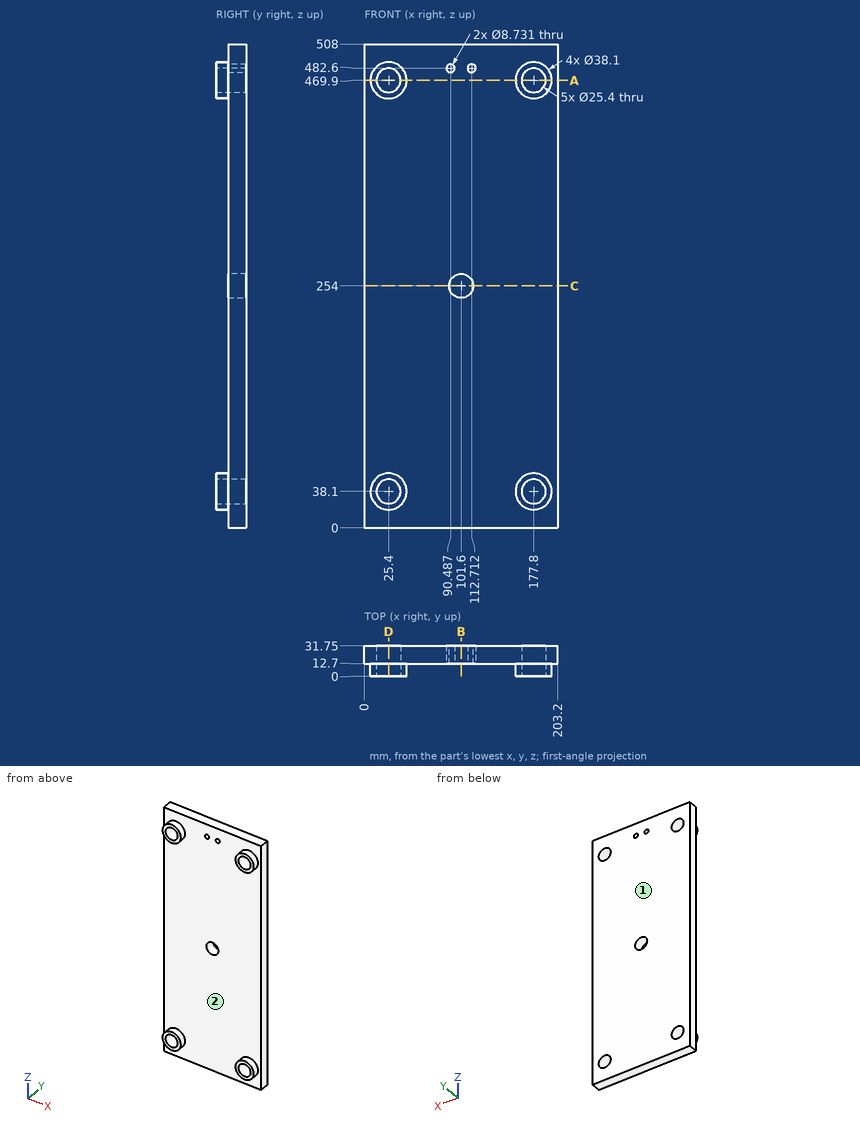
The drawing under review shows one solid part. Ordinate dimensions are in mm from its lowest x, y, z. Round coordinates to 2 decimals unless told otherwise and drop trailing zeros. Loops run counter-clockwise (first coordinate to the right, second up) from the corner with the lowest first, then second, coordinate; pieces in that order, holes last. Notation, with made-up numbers: (-39.75, 11.5) - (-3.75, 11.5) arc R24 cw to (-3.75, 27.5) - close; hole circle Ø11 at (85.25, 67.5). An arc over 180 degrees is marked (long way). One line per question, with ' | ' between items.
1. We need section D-D, the plane x = 25.4. State the section outline as (y, z) points, and give its area (3 significant figures).
Results are:
outline: (0, 19.05) - (12.7, 19.05) - (12.7, 0) - (31.75, 0) - (31.75, 25.4) - (0, 25.4) - close; (0, 50.8) - (31.75, 50.8) - (31.75, 457.2) - (0, 457.2) - (0, 450.85) - (12.7, 450.85) - (12.7, 57.15) - (0, 57.15) - close; (0, 482.6) - (31.75, 482.6) - (31.75, 508) - (12.7, 508) - (12.7, 488.95) - (0, 488.95) - close | area: 9,030 mm²
2. We need section A-A, the plane z = 469.9. State the section outline as (x, y) points.
Results are:
outline: (0, 12.7) - (6.35, 12.7) - (6.35, 0) - (12.7, 0) - (12.7, 31.75) - (0, 31.75) - close; (38.1, 0) - (44.45, 0) - (44.45, 12.7) - (158.75, 12.7) - (158.75, 0) - (165.1, 0) - (165.1, 31.75) - (38.1, 31.75) - close; (190.5, 0) - (196.85, 0) - (196.85, 12.7) - (203.2, 12.7) - (203.2, 31.75) - (190.5, 31.75) - close
3. We need section B-B, the plane x = 101.6. State the section outline as (y, z) points.
Results are:
outline: (12.7, 0) - (31.75, 0) - (31.75, 241.3) - (12.7, 241.3) - close; (12.7, 266.7) - (31.75, 266.7) - (31.75, 508) - (12.7, 508) - close
4. We need section C-C, the plane z = 254. State the section outline as (x, y) points, and give its area (3 significant figures).
Results are:
outline: (0, 12.7) - (88.9, 12.7) - (88.9, 31.75) - (0, 31.75) - close; (114.3, 12.7) - (203.2, 12.7) - (203.2, 31.75) - (114.3, 31.75) - close | area: 3,390 mm²
5. Draft analysis for pull direction Z (two halves, no side actions). For the marked faces 1 and 2, state which applies: released by +Z, released by -Z, zero draft, split by the parting line, or undercut.
Results are:
face 1: zero draft | face 2: undercut
6. Clearance check with flat-ended pins moving along their axes: P1, Ø10, axis at x = 149.5, z = 201.5, coming from the -Y side; P2, Ø23, axis at x = 25.4, z = 469.9, coming from the +Y side; P3, Ø1, axis at x = 178.5, y = 10, coming from the +Z side. State where each tip first meets the part, or that it passes through.
Results are:
P1: stops at y = 12.7 | P2: passes through | P3: stops at z = 488.95
7. For L1, parallel to X at y = 13, z = 469.9; L2, parallel to Y at x = 131.5, z = 169; L3, parallel to Z at x = 112, y = 26 (1 decimal), list the stretches that pass through material, from the lowest coordinate up. Write a range as [from, to].
Results are:
L1: x = [0, 12.7], [38.1, 165.1], [190.5, 203.2] | L2: y = [12.7, 31.75] | L3: z = [0, 246.7], [261.3, 478.3], [486.9, 508]
